Model file for the job. Use its own axes, mm. A direction names the side the tool comes from. Coordinates: 2 decimals unless noted, no trailing zeros. Loops run counter-clockwise (first coordinate to the right, second up) from the corner with the lowest first, then second, coordinate; pieces in that order, holes last.
from build123d import *

# Parameters (mm, degrees)
SKETCH1_R           = 1.725
SKETCH1_R_2         = 13.1
SKETCH1_W           = 23.65
SKETCH1_H           = 42.25
BOSS_EXTRUDE1_DEPTH = 5.1
CUT_EXTRUDE1_START  = -2
SKETCH2_R           = 1.725
CUT_EXTRUDE1_DEPTH  = 2
FILLET1_R           = 4
FILLET2_R           = 20
FILLET3_R           = 15
FILLET4_R           = 1


with BuildPart() as part:
    # Sketch1 → Boss-Extrude1 (new body)
    with BuildSketch(Plane.XY):
        Polygon((12.6125, 29), (12.6125, 21.5), (-21.2125, 21.5), (-21.2125, -21.5), (12.6125, -21.5), (12.6125, -29), (44.6125, -29), (44.6125, 29), align=None)
        with Locations((-15, -8)):
            Circle(SKETCH1_R, mode=Mode.SUBTRACT)
        with Locations((-15, 8)):
            Circle(SKETCH1_R, mode=Mode.SUBTRACT)
        with Locations((11, 12)):
            Circle(SKETCH1_R, mode=Mode.SUBTRACT)
        with Locations((11, -12)):
            Circle(SKETCH1_R, mode=Mode.SUBTRACT)
        Circle(SKETCH1_R_2, mode=Mode.SUBTRACT)
        with BuildLine():
            Line((22.229319933, 27.275), (25.229319933, 27.275))
            ThreePointArc((25.229319933, 27.275), (26.954319933, 25.55), (25.229319933, 23.825))
            Line((25.229319933, 23.825), (22.229319933, 23.825))
            ThreePointArc((22.229319933, 23.825), (20.504319933, 25.55), (22.229319933, 27.275))
        make_face(mode=Mode.SUBTRACT)
        with BuildLine():
            Line((32.029319933, 27.275), (35.029319933, 27.275))
            ThreePointArc((35.029319933, 27.275), (36.754319933, 25.55), (35.029319933, 23.825))
            Line((35.029319933, 23.825), (32.029319933, 23.825))
            ThreePointArc((32.029319933, 23.825), (30.304319933, 25.55), (32.029319933, 27.275))
        make_face(mode=Mode.SUBTRACT)
        with BuildLine():
            Line((22.229319933, -23.825), (25.229319933, -23.825))
            ThreePointArc((25.229319933, -23.825), (26.954319933, -25.55), (25.229319933, -27.275))
            Line((25.229319933, -27.275), (22.229319933, -27.275))
            ThreePointArc((22.229319933, -27.275), (20.504319933, -25.55), (22.229319933, -23.825))
        make_face(mode=Mode.SUBTRACT)
        with BuildLine():
            Line((32.029319933, -23.825), (35.029319933, -23.825))
            ThreePointArc((35.029319933, -23.825), (36.754319933, -25.55), (35.029319933, -27.275))
            Line((35.029319933, -27.275), (32.029319933, -27.275))
            ThreePointArc((32.029319933, -27.275), (30.304319933, -25.55), (32.029319933, -23.825))
        make_face(mode=Mode.SUBTRACT)
        with Locations((28.6125, 0)):
            Rectangle(SKETCH1_W, SKETCH1_H, mode=Mode.SUBTRACT)
    extrude(amount=BOSS_EXTRUDE1_DEPTH)

    # Sketch2 → Cut-Extrude1 (cut)
    with BuildSketch(Plane.XY.offset(5.1).offset(CUT_EXTRUDE1_START)):
        with BuildLine():
            Line((6.7875, 11.204456424), (6.7875, 21.5))
            Line((6.7875, 21.5), (-21.2125, 21.5))
            Line((-21.2125, 21.5), (-21.2125, -21.5))
            Line((-21.2125, -21.5), (6.7875, -21.5))
            Line((6.7875, -21.5), (6.7875, -11.204456424))
            ThreePointArc((6.7875, -11.204456424), (-13.1, 0), (6.7875, 11.204456424))
        make_face()
        with Locations((-15, -8)):
            Circle(SKETCH2_R, mode=Mode.SUBTRACT)
        with Locations((-15, 8)):
            Circle(SKETCH2_R, mode=Mode.SUBTRACT)
    extrude(amount=CUT_EXTRUDE1_DEPTH, mode=Mode.SUBTRACT)

    # Fillet1
    fillet1_edges = [part.edges().sort_by_distance(p)[0] for p in [
        (12.6125, 29, 2.55),
        (44.6125, 29, 2.55),
        (44.6125, -29, 2.55),
        (12.6125, -29, 2.55),
    ]]
    fillet(fillet1_edges, radius=FILLET1_R)

    # Fillet2
    fillet2_edges = [part.edges().sort_by_distance(p)[0] for p in [
        (-21.2125, -21.5, 1.55),
        (-21.2125, 21.5, 1.55),
    ]]
    fillet(fillet2_edges, radius=FILLET2_R)

    # Fillet3
    # the kernel refuses this fillet: 15 mm, written as the material it adds along each edge
    with BuildSketch(Plane(origin=(6.7875, -21.5, 3.1), x_dir=(-1, 0, 0), z_dir=(0, 1, 0))) as fillet3_piece_1_section:
        with BuildLine():
            CenterArc((7.483314774, 15), FILLET3_R, 240.073565133, 29.926434867)
            Line((0, 2), (-0.149666295, 1.74))
            ThreePointArc((-0.149666295, 1.74), (-0.3, 1), (-0.3, 0))
            Line((-0.3, 0), (0, -0.3))
            Line((0, -0.3), (7.483314774, -0.3))
            Line((7.483314774, -0.3), (7.483314774, 0))
        make_face()
    fillet3_piece_1 = extrude(amount=29.00383051, mode=Mode.PRIVATE)
    fillet3_piece_1 = fillet3_piece_1 - Plane(origin=(0, 0, 3.507090061), x_dir=(1, 0, 0), z_dir=(0, 0, -1)) * Cylinder(13.1, 88, mode=Mode.PRIVATE)
    add(fillet3_piece_1)
    with BuildSketch(Plane(origin=(6.7875, -7.50383051, 3.1), x_dir=(-1, 0, 0), z_dir=(0, 1, 0))) as fillet3_piece_2_section:
        with BuildLine():
            CenterArc((7.483314774, 15), FILLET3_R, 240.073565133, 29.926434867)
            Line((0, 2), (-0.149666295, 1.74))
            ThreePointArc((-0.149666295, 1.74), (-0.3, 1), (-0.3, 0))
            Line((-0.3, 0), (0, -0.3))
            Line((0, -0.3), (7.483314774, -0.3))
            Line((7.483314774, -0.3), (7.483314774, 0))
        make_face()
    fillet3_piece_2 = extrude(amount=29.00383051, mode=Mode.PRIVATE)
    fillet3_piece_2 = fillet3_piece_2 - Plane(origin=(0, 0, 3.507090028), x_dir=(1, 0, 0), z_dir=(0, 0, -1)) * Cylinder(13.1, 88, mode=Mode.PRIVATE)
    add(fillet3_piece_2)

    # Fillet4
    # the kernel refuses this fillet: 1 mm, written as the material it takes off along each edge
    with BuildSketch(Plane(origin=(4.2875, -21.5, 5.1), x_dir=(0, 1, 0), z_dir=(1, 0, 0)), Plane(origin=(12.6125, 21.5, 5.1), x_dir=(0, -1, 0), z_dir=(-1, 0, 0))) as fillet4_piece_1:
        with BuildLine():
            CenterArc((FILLET4_R, -FILLET4_R), FILLET4_R, 90, 90)
            Line((0, -FILLET4_R), (0, 0))
            Line((0, 0), (FILLET4_R, 0))
        make_face()
    extrude(amount=8.325, mode=Mode.SUBTRACT)
    with BuildSketch(Plane(origin=(-1.2125, -21.5, 3.1), x_dir=(0, 1, 0), z_dir=(1, 0, 0)), Plane(origin=(-0.695814774, 21.5, 3.1), x_dir=(0, -1, 0), z_dir=(-1, 0, 0))) as fillet4_piece_2:
        with BuildLine():
            CenterArc((FILLET4_R, -FILLET4_R), FILLET4_R, 90, 90)
            Line((0, -FILLET4_R), (0, 0))
            Line((0, 0), (FILLET4_R, 0))
        make_face()
    extrude(amount=0.516685226, mode=Mode.SUBTRACT)
    with BuildSketch(Plane(origin=(-21.2125, 1.5, 3.1), x_dir=(1, 0, 0), z_dir=(0, -1, 0))) as fillet4_piece_3:
        with BuildLine():
            CenterArc((FILLET4_R, -FILLET4_R), FILLET4_R, 90, 90)
            Line((0, -FILLET4_R), (0, 0))
            Line((0, 0), (FILLET4_R, 0))
        make_face()
    extrude(amount=3, mode=Mode.SUBTRACT)
    with BuildSketch(Plane(origin=(-1.2125, 1.5, 3.1), x_dir=(0, 1, 0), z_dir=(1, 0, 0))) as fillet4_piece_4:
        with BuildLine():
            CenterArc((20 - FILLET4_R, -FILLET4_R), FILLET4_R, 0, 90)
            Line((20, -FILLET4_R), (20, 0))
            Line((20, 0), (20 - FILLET4_R, 0))
        make_face()
    revolve(axis=Axis((-1.2125, 1.5, 3.1), (0, 0, 1)), revolution_arc=90, mode=Mode.SUBTRACT)
    with BuildSketch(Plane(origin=(-1.2125, -1.5, 3.1), x_dir=(-1, 0, 0), z_dir=(0, 1, 0))) as fillet4_piece_5:
        with BuildLine():
            CenterArc((20 - FILLET4_R, -FILLET4_R), FILLET4_R, 0, 90)
            Line((20, -FILLET4_R), (20, 0))
            Line((20, 0), (20 - FILLET4_R, 0))
        make_face()
    revolve(axis=Axis((-1.2125, -1.5, 3.1), (0, 0, 1)), revolution_arc=90, mode=Mode.SUBTRACT)
    with BuildSketch(Plane(origin=(-0.695814774, -21.5, 18.1), x_dir=(0.6357570418169636, 0, -0.7718892302527245), z_dir=(0.7718892302527245, 0, 0.6357570418169636))) as fillet4_piece_6:
        with BuildLine():
            CenterArc((15 + FILLET4_R, FILLET4_R), FILLET4_R, 180, 90)
            Line((15 + FILLET4_R, 0), (15, 0))
            Line((15, 0), (15, FILLET4_R))
        make_face()
    revolve(axis=Axis((-0.695814774, -21.5, 18.1), (0, 1, 0)), revolution_arc=39.476155484, mode=Mode.SUBTRACT)
    with BuildSketch(Plane(origin=(-0.695814774, 21.5, 18.1), x_dir=(0.6357570418169636, 0, -0.7718892302527245), z_dir=(0.7718892302527245, 0, 0.6357570418169636))) as fillet4_piece_7:
        with BuildLine():
            CenterArc((15 + FILLET4_R, -FILLET4_R), FILLET4_R, 90, 90)
            Line((15 + FILLET4_R, 0), (15, 0))
            Line((15, 0), (15, -FILLET4_R))
        make_face()
    revolve(axis=Axis((-0.695814774, 21.5, 18.1), (0, 1, 0)), revolution_arc=39.476155484, mode=Mode.SUBTRACT)


solid = part.part
Q1. Slice it at C-C (x = 11). List the corners of the cut face in (y, z) (3 decimals).
Answers:
outline: (-21.5, 0) - (-13.725, 0) - (-13.725, 5.1) - (-20.5, 5.1) arc R1 ccw to (-21.5, 4.1) - close; (-10.275, 0) - (-7.114, 0) - (-7.114, 5.1) - (-10.275, 5.1) - close; (7.114, 0) - (10.275, 0) - (10.275, 5.1) - (7.114, 5.1) - close; (13.725, 0) - (21.5, 0) - (21.5, 4.1) arc R1 ccw to (20.5, 5.1) - (13.725, 5.1) - close
Q2. Slice it at A-A (x = 39.5). List the corners of the cut face in (y, z) (3 decimals).
Answers:
outline: (-29, 0) - (-21.125, 0) - (-21.125, 5.1) - (-29, 5.1) - close; (21.125, 0) - (29, 0) - (29, 5.1) - (21.125, 5.1) - close
Q3. Which spindle directions (+Z, -Z, +X, -X, +Y, -Y) get a long thin tool onto all of the face, cutting with end or side? Do faces 5 (the flat face through (34, -27.275, 3)), 6 (the flat face through (-15, 0, 3.1)), 7 (the cylindrical face through (13.815, -27.859, 2.586)). Say none if no direction does.
Answers:
face 5: +Z, -Z
face 6: +Z, -X, +Y, -Y
face 7: +Z, -Z, -X, -Y
Q4. Slice it at B-B (y = 0). List the corners of the cut face in (x, z), and give its area (3 significant figures).
Answers:
outline: (-21.21, 0) - (-13.1, 0) - (-13.1, 3.1) - (-20.21, 3.1) arc R1 ccw to (-21.21, 2.1) - close; (13.1, 0) - (16.79, 0) - (16.79, 5.1) - (13.1, 5.1) - close; (40.44, 0) - (44.61, 0) - (44.61, 5.1) - (40.44, 5.1) - close
area: 65.0 mm2
Q5. Slice it at D-D (z = 1). Count the separate pieces of the cut face and the enclosed holes in it, and give its area (3 significant figures).
Answers:
separate pieces: 1
enclosed holes: 10
area: 1,470 mm2
Q6. Mould opens along X. For faces 1 (the flat face through (29, 29, 3)), 2 (the cylindrical face through (3.23, -16.95, 3.623)), 3 (the flat face through (24, -23.825, 3)), 4 (the flat face through (28, 21.125, 3)) say: +X half, -X half, draft (parallel to the pull), parting line (faces both ways), or undercut.
Answers:
face 1: draft
face 2: -X half
face 3: undercut
face 4: undercut
Q7. Flat gauge pins, fed straight in: P1, Ø21.5, axis at x = -14.5, y = -4.5, coming from the +Z side; P2, Ø1, axis at y = -23.5, z = 2.5, coming from the -X side; P3, Ø2.5, axis at y = -2.5, z = 2, coming from the -X side; P4, Ø2, axis at y = -6, z = 2.5, coming from the -X side. Where does each tip first touch, or does it go through?
Answers:
P1: stops at z = 3.1
P2: stops at x = 12.61
P3: stops at x = -21.21
P4: stops at x = -20.89
Q8. Drill centre lines: line 1 (Y direction, x = 37, z = 0.35) (3 decimals); line 2 (Y direction, x = 11, z = 4) (3 decimals); line 3 (X direction, y = 0, z = 3.55). Where is each one in solid material? Low to high.
Answers:
line 1: y = -29 to -21.125, 21.125 to 29
line 2: y = -21.5 to -13.725, -10.275 to -7.114, 7.114 to 10.275, 13.725 to 21.5
line 3: x = 13.1 to 16.79, 40.44 to 44.61
